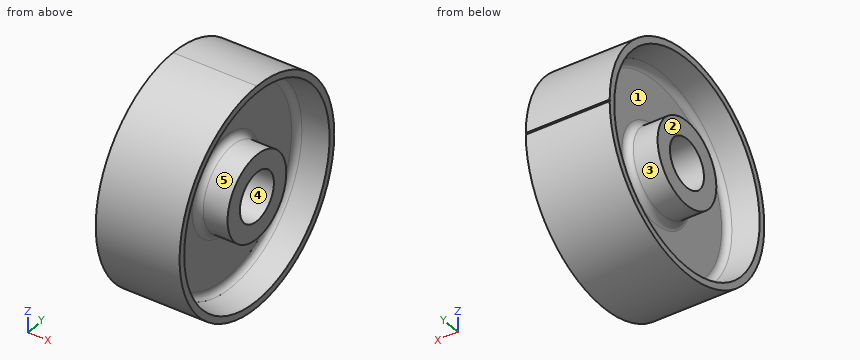
```python
from build123d import *

# Parameters (mm, degrees)
FILLET_1_R          = 3
CUT_EXTRUDE_1_DEPTH = 81.274528962


with BuildPart() as part:
    # 草圖1 → 旋轉1 (revolve)
    with BuildSketch(Plane.XY, mode=Mode.PRIVATE) as revolve_1_sk:
        Polygon((-19, 11), (19, 11), (19, 19), (5, 19), (5, 45), (19, 47), (19, 50), (-19, 50), (-19, 47), (-5, 45), (-5, 19), (-19, 19), align=None)
    revolve(revolve_1_sk.sketch.rotate(Axis((-30.665853659, 0, 0), (1, 0, 0)), 90), axis=Axis((-30.665853659, 0, 0), (1, 0, 0)))

    # 圓角1
    fillet_1_edges = [part.edges().sort_by_distance(p)[0] for p in [
        (-5, 0, -19),
        (5, 0, -19),
        (5, 0, -45),
        (-5, 0, -45),
    ]]
    fillet(fillet_1_edges, radius=FILLET_1_R)

    # 草圖2 → 伸長1 (cut, through all)
    with BuildSketch(Plane(origin=(19, 0, 0), x_dir=(0, 0, -1), z_dir=(1, 0, 0))):
        Polygon((-0.913442032, 50.94560231), (0.913442032, 50.94560231), (0, 49.363474301), align=None)
    extrude(amount=-CUT_EXTRUDE_1_DEPTH, mode=Mode.SUBTRACT)


solid = part.part
```
Input: part model. Units: mm. Frame: model coordinates. Face numbers are marked on the shaded views. A direction names the side the tool comes from. Round coordinates to 2 decimals unless told otherwise and drop trailing zeros. Order: outer loops, then holes, each group sorted by start corner. A loop starts at its lowest first (then second) coordinate and runs counter-clockwise, first axis right, second up. Notation, with made-up numbers: (34, 81) - (71, 81) arc R22 ccw to (71, 87) - close; hole circle Ø2 at (77.5, 69). An arc over 180 degrees is marked (long way). One line per question, with ' | ' between items. Start each with the question number.
1) Cut plane A-A, the plane x = 12. Return the cut outline in (y, z).
2) Set-up query: the marked faces 3, 4 and 5. Return all of +Z, -Z, +X, -X, +Y, -Y with unobstructed straight access to the full face (end or side cutting, diameter ignored); none if empty.
3) Cut plane B-B, the plane x = 17.5. Return the cut outline in (y, z), then the cut area to 3 significant figures.
4) Ray query, probe 1 along Z at (x, y) = (14, -6); probe 2 along X at (y, z) = (20, -26.5); probe 3 along Y at (x, z) = (-16.5, -27). Return the intervals inside material, ascending.
5) Contact query for flat-ended pins moving along their axis: P1, Ø10, axis at x = -10.5, y = -10, coming from the +Z side; P2, Ø1, axis at x = -7, y = -36, coming from the -Z side; P3, Ø8, axis at x = -6.5, z = 34.5, coming from the -Y side. Output: stop coordinate, or through.
6) Pull-direction query (Z, two-part tool) for the marked faces 1 and 2; classes: +Z half, -Z half, draft (parallel to the pull), parting line (faces both ways), or undercut.
Worked out:
1) outline: circle Ø38 at (0, 0); (49.36, 0) - (50, 0.37) arc R50 ccw (long way) to (50, -0.37) - close; hole circle Ø92 at (0, 0); hole circle Ø22 at (0, 0)
2) face 3: -X | face 4: +X, -X | face 5: +X
3) outline: circle Ø38 at (0, 0); (49.36, 0) - (50, 0.37) arc R50 ccw (long way) to (50, -0.37) - close; hole circle Ø93.57 at (0, 0); hole circle Ø22 at (0, 0) | area: 1,730 mm^2
4) probe 1: z = -49.64 to -45.9, -18.03 to -9.22, 9.22 to 18.03, 45.9 to 49.64 | probe 2: x = -5 to 5 | probe 3: y = -42.08 to -38.03, 38.03 to 42.08
5) P1: stops at z = 49.75 | P2: stops at z = -35.21 | P3: stops at y = -39.62
6) face 1: undercut | face 2: draft
